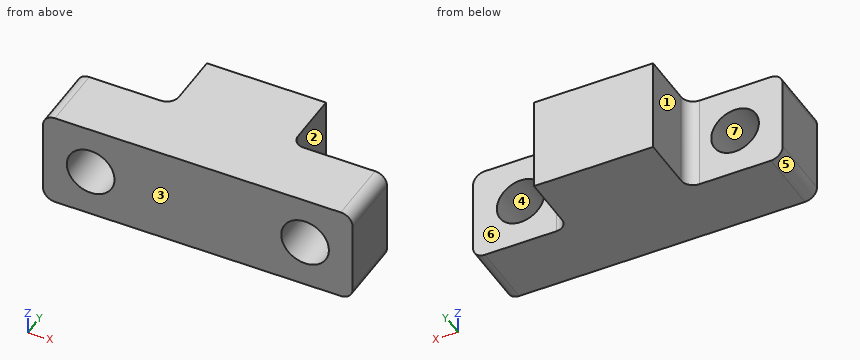
Autodesk Inventor part; units mm, degrees
ref_plane "YZ Plane" through (0, 0, 0) normal (1, 0, 0) x (0, 1, 0)
ref_plane "XZ Plane" through (0, 0, 0) normal (0, 1, 0) x (-1, 0, 0)
ref_plane "XY Plane" through (0, 0, 0) normal (0, 0, 1) x (1, 0, 0)
sketch "Sketch1" plane through (0, 0, 0) normal (0, 0, 1) x (1, 0, 0)
  line L0 (0, -14.2875) -> (0, 20.6375)
  line L1 (0, 20.6375) -> (-15.875, 20.6375)
  line L2 (-15.875, 20.6375) -> (-15.875, 3.175)
  line L3 (-15.875, 3.175) -> (-41.275, 3.175)
  line L4 (-41.275, 3.175) -> (-41.275, -14.2875)
  line L5 (-41.275, -14.2875) -> (0, -14.2875)
extrude "Extrusion1" add sketch "Sketch1" along normal blind 25.4
sketch "Sketch2" plane through (-41.275, 3.175, 0) normal (0, 1, 0) x (1, 0, 0)
  circle A0 centre (12.7, -12.7) radius 6.35
extrude "Extrusion2" cut sketch "Sketch2" against normal through all
fillet "Fillet1" radius 3.175 3 edges at (-41.275, -5.5563, 25.4) (-41.275, -5.5563, 0) (-15.875, 3.175, 12.7)
mirror "Mirror1" about plane through (0, 20.6375, 0) normal (1, 0, 0) of "Extrusion1", "Extrusion2", "Fillet1"
properties part number "Left half"
Verification items for the finished model (mm, model axes). Face numbers are marked on the shaded views. A direction names the side the tool comes from. Coordinates: 2 decimals unless noted, no trailing zeros. Write each loop counter-clockwise with the first axis right and the second up, starting at its lowest first coordinate (ties: lowest second). Pieces come first, ordered by that corner, then holes. Notation, with made-up numbers: (34, 7.5) - (90, 7.5) arc R12 cw to (90, 29.5) - close; hole circle Ø9 at (-10, 74.25). An arc over 180 degrees is marked (long way). One line per question, with ' | ' between items. Start each with the question number.
1. Section check A-A (z = 12.7). Count the separate pieces of the cut face and the enclosed holes in it, plus the area to 3 significant figures.
2. Gauge pin test, flat ends, axial feed: P1, Ø5, axis at x = 31.5, z = 20, coming from the +Y side (3 decimals); P2, Ø7, axis at y = 13, z = 10.5, coming from the -X side (3 decimals); P3, Ø7, axis at y = 14, z = 18, coming from the +X side (3 decimals). Record the tip position at first contact, or that the pin passes through.
3. Material ranges on line 1 along X through (y, z) = (-2, 12.7) (3 decimals); line 2 along X through (y, z) = (-12, 14.75) (3 decimals); line 3 along Z through (x, y) = (33.5, 2.5), recorded low to high.
4. Section check B-B (y = -3). Enter the section's corners in (x, z) (3 decimals).
5. Section check C-C (x = 29). Enter the section's corners in (y, z) (1 decimal), plus the area to 3 significant figures.
6. Draft check along X on the marked faces 4, 5, 6 and 7. Enter one of: released by +X, released by -X, zero draft, split by the parting line, or undercut.
7. Access from +Z, -Z, +X, -X, +Y, -Y to the whole of each face (thin tool, end or side, straight path). Record for the marked faces 1, 2 and 3.
Computed values:
1) separate pieces: 3 | enclosed holes: 0 | area: 1,560 mm²
2) P1: y = 3.175 | P2: x = -15.875 | P3: x = 15.875
3) line 1: -41.275 to -34.925, -22.225 to 22.225, 34.925 to 41.275 | line 2: -41.275 to -34.585, -22.565 to 22.565, 34.585 to 41.275 | line 3: 0 to 8.69, 16.71 to 25.4
4) outline: (-41.275, 3.175) arc R3.175 ccw to (-38.1, 0) - (38.1, 0) arc R3.175 ccw to (41.275, 3.175) - (41.275, 22.225) arc R3.175 ccw to (38.1, 25.4) - (-38.1, 25.4) arc R3.175 ccw to (-41.275, 22.225) - close; hole circle Ø12.7 at (-28.575, 12.7); hole circle Ø12.7 at (28.575, 12.7)
5) outline: (-14.3, 0) - (3.2, 0) - (3.2, 6.4) - (-14.3, 6.4) - close; (-14.3, 19) - (3.2, 19) - (3.2, 25.4) - (-14.3, 25.4) - close | area: 222 mm²
6) face 4: undercut | face 5: released by -X | face 6: zero draft | face 7: undercut
7) face 1: +Z, -Z, -X, +Y | face 2: +Z, -Z, +X, +Y | face 3: +Z, -Z, +X, -X, -Y
